from build123d import *

# Parameters (mm, degrees)
SKETCH1_R           = 1.75
BOSS_EXTRUDE1_DEPTH = 5
FILLET1_R           = 1
SKETCH2_R           = 3.1
CUT_EXTRUDE1_DEPTH  = 3
SKETCH3_W           = 83.675621306
SKETCH3_H           = 27.808708761
CUT_EXTRUDE2_DEPTH  = 5


with BuildPart() as part:
    # Sketch1 → Boss-Extrude1 (new body)
    with BuildSketch(Plane(origin=(0, 0, 0), x_dir=(1, 0, 0), z_dir=(0, 1, 0))):
        with BuildLine():
            ThreePointArc((-29.5, 4), (-33.5, 0), (-29.5, -4))
            ThreePointArc((-29.5, -4), (-16.900654795, -5.373538993), (-4.893229568, -9.429626812))
            ThreePointArc((-4.893229568, -9.429626812), (14.756477238, -11.986867848), (32.328427125, -2.828427125))
            ThreePointArc((32.328427125, -2.828427125), (32.328427125, 2.828427125), (26.671572875, 2.828427125))
            ThreePointArc((26.671572875, 2.828427125), (13.359489628, -4.109785544), (-1.526651892, -2.172481729))
            ThreePointArc((-1.526651892, -2.172481729), (-15.176874162, 2.438540137), (-29.5, 4))
        make_face()
        with Locations(Location((-29.5, 0, 0), (0, 0, 270))):
            Circle(SKETCH1_R, mode=Mode.SUBTRACT)
        with Locations(Location((29.5, 0, 0), (0, 0, 270))):
            Circle(SKETCH1_R, mode=Mode.SUBTRACT)
    extrude(amount=BOSS_EXTRUDE1_DEPTH)

    # Fillet1
    fillet1_edges = [part.edges().sort_by_distance(p)[0] for p in [
        (-16.900654795, 5, 5.373538993),
        (14.756477238, 5, 11.986867848),
        (32.328427125, 5, -2.828427125),
        (13.359489628, 5, 4.109785544),
        (-15.176874162, 5, -2.438540137),
        (13.359489628, 0, 4.109785544),
        (32.328427125, 0, -2.828427125),
        (14.756477238, 0, 11.986867848),
        (-16.900654795, 0, 5.373538993),
        (-33.5, 0, 0),
        (-15.176874162, 0, -2.438540137),
        (-33.5, 5, 0),
    ]]
    fillet(fillet1_edges, radius=FILLET1_R)

    # Sketch2 → Cut-Extrude1 (cut)
    with BuildSketch(Plane.XZ):
        with Locations(Location((29.5, 0, 0), (0, 0, 270))):
            Circle(SKETCH2_R)
        with Locations(Location((-29.5, 0, 0), (0, 0, 270))):
            Circle(SKETCH2_R)
    extrude(amount=-CUT_EXTRUDE1_DEPTH, mode=Mode.SUBTRACT)


with BuildPart() as body_2:
    # Mirror1: mirrored copy
    add(part.part.mirror(Plane(origin=(0, -10, 0), x_dir=(0, 0, 1), z_dir=(0, -1, 0))))


with BuildPart() as part_1:
    add(part.part)

    # Sketch3 → Cut-Extrude2 (cut)
    with BuildSketch(Plane.XZ):
        with Locations((4.363579438, 1.855920518)):
            Rectangle(SKETCH3_W, SKETCH3_H)
    extrude(amount=-CUT_EXTRUDE2_DEPTH, mode=Mode.SUBTRACT)


solid = body_2.part
Can you work these out from the model? Positions are in its coordinate system, mm. A direction names the side the tool comes from. Round coordinates to 2 decimals unless told otherwise and drop trailing zeros. Answer in a Markdown table with one row per item.
(1) Suppose I cut it at A-A, the plane z = 0. Count the separate pieces of the cut face and the enclosed holes in it, plus the area to 3 significant figures.
From the geometry:
| item | result |
|---|---|
| separate pieces | 4 |
| enclosed holes | 0 |
| area | 130 mm2 |
(2) Which directions (+Z, -Z, +X, -X, +Y, -Y) give clear straight access to the entire face, cutting with the end or side of a thin tool? Please do faces 1 (the face through (32.39, -22.479, -2.766)), 2 (the face through (-26.426, -21.479, 0.404)), 3 (the face through (-15, -22.5, -2.4)).
From the geometry:
| item | result |
|---|---|
| face 1 | +Y, -Y |
| face 2 | +Y |
| face 3 | -Z, +Y, -Y |
(3) If we mould it in two halves opening along Z, with no side actions, what happens to faces 4 (the face through (32.574, -21.479, 0.404)), 5 (the face through (-33.5, -22.5, -0.1)), 6 (the face through (-17.074, -22.479, 5.335))? For each: released by +Z, released by -Z, zero draft, split by the parting line, or undercut.
From the geometry:
| item | result |
|---|---|
| face 4 | undercut |
| face 5 | split by the parting line |
| face 6 | released by +Z |
(4) Please list where these lines run through material, in increasing order: L1, parallel to Z at x = -29.5, y = -21.8; L2, parallel to Z at x = -27, y = -21.25; L3, parallel to X at y = -22.75, z = 8.5. Write a range as from..to.
From the geometry:
| item | result |
|---|---|
| L1 | z = -4..-3.1, 3.1..4 |
| L2 | z = -3.95..-1.83, 1.83..4.05 |
| L3 | x = -7.01..24.73 |
(5) For P1, Ø5.5, axis at x = -29.5, z = 0, coming from the +Y side; P2, Ø3, axis at y = -22.5, z = 7, coming from the +X side; P3, Ø5, axis at x = 30.5, z = 0, coming from the +Y side (3 decimals), each with a flat end and sliding along its axis, tell me the tip position at first contact or that it passes through.
From the geometry:
| item | result |
|---|---|
| P1 | stops at y = -23 |
| P2 | stops at x = 29.31 |
| P3 | stops at y = -20.005 |
